from build123d import *

# Parameters (mm, degrees)
BOSS_EXTRUDE1_DEPTH   = 32
BOSS_EXTRUDE1_2_DEPTH = 32
BOSS_EXTRUDE2_DEPTH   = 72
CUT_EXTRUDE1_REACH    = 135.547
CUT_EXTRUDE2_REACH    = 168.292
SKETCH3_R             = 10


with BuildPart() as part:
    # Sketch1 → Boss-Extrude1 (new body)
    with BuildSketch(Plane.XY):
        Polygon((0, 42.5), (1.56434465, 52.376883406), (120.39128367, 33.556545174), (75, 85), (0, 85), align=None)
    extrude(amount=BOSS_EXTRUDE1_DEPTH)



with BuildPart() as body_2:
    # Sketch1 → Boss-Extrude1 2 (new body)
    with BuildSketch(Plane.XY):
        Polygon((150, 0), (120.39128367, 33.556545174), (118.82693902, 23.679661768), (0, 42.5), (0, 0), align=None)
    extrude(amount=BOSS_EXTRUDE1_2_DEPTH)


with BuildPart() as part_1:
    add(part.part)

    add(body_2.part)  # Boss-Extrude2 merges body 2
    # Sketch1<4> → Boss-Extrude2 (add)
    with BuildSketch(Plane.XY):
        Polygon((0, 42.5), (1.56434465, 52.376883406), (120.39128367, 33.556545174), (118.82693902, 23.679661768), align=None)
    extrude(amount=BOSS_EXTRUDE2_DEPTH)

    # Cut-Extrude1: up to this plane
    cut_extrude1_end = Plane(origin=(0, 0, 32), z_dir=(0, 1, 0))
    # Sketch2 → Cut-Extrude1 (cut, up to the surface)
    with BuildSketch(Plane(origin=(84.338521401, 74.416342412, 0), x_dir=(0, 0, -1), z_dir=(0.7498378553650925, 0.6616216370868464, 0)), mode=Mode.PRIVATE) as cut_extrude1_sk1:
        Polygon((0, -22.564325319), (-8, -22.564325319), (-8, -12.564325319), (-24, -12.564325319), (-24, -72.564325319), (-8, -72.564325319), (-8, -62.564325319), (0, -62.564325319), align=None)
    cut_extrude1_tool1 = split(extrude(cut_extrude1_sk1.sketch, amount=-CUT_EXTRUDE1_REACH, mode=Mode.PRIVATE), bisect_by=cut_extrude1_end, keep=Keep.BOTH, mode=Mode.PRIVATE)
    add(cut_extrude1_tool1.solids().sort_by_distance((112.5, 42.5, 13))[0], mode=Mode.SUBTRACT)

    # Sketch3 → Cut-Extrude2 (cut, up to next)
    with BuildSketch(Plane(origin=(6.56661113, 41.459950971, 0), x_dir=(0.9876883405951378, -0.1564344650402311, 0), z_dir=(-0.1564344650402311, -0.9876883405951378, 0)), mode=Mode.PRIVATE) as cut_extrude2_sk1:
        with Locations((43.351535236, 54)):
            Circle(SKETCH3_R)
    cut_extrude2_tool1 = extrude(cut_extrude2_sk1.sketch, amount=-CUT_EXTRUDE2_REACH, mode=Mode.PRIVATE) & part_1.part
    # Sketch3 → Cut-Extrude2 (cut, up to next)
    with BuildSketch(Plane(origin=(6.56661113, 41.459950971, 0), x_dir=(0.9876883405951378, -0.1564344650402311, 0), z_dir=(-0.1564344650402311, -0.9876883405951378, 0)), mode=Mode.PRIVATE) as cut_extrude2_sk2:
        Polygon((113.659666997, 72), (88.659666997, 72), (113.659666997, 47), align=None)
    cut_extrude2_tool2 = extrude(cut_extrude2_sk2.sketch, amount=-CUT_EXTRUDE2_REACH, mode=Mode.PRIVATE) & part_1.part
    # Sketch3 → Cut-Extrude2 (cut, up to next)
    with BuildSketch(Plane(origin=(6.56661113, 41.459950971, 0), x_dir=(0.9876883405951378, -0.1564344650402311, 0), z_dir=(-0.1564344650402311, -0.9876883405951378, 0)), mode=Mode.PRIVATE) as cut_extrude2_sk3:
        Polygon((-6.648464764, 72), (-6.648464764, 32), (16.445546003, 72), align=None)
    cut_extrude2_tool3 = extrude(cut_extrude2_sk3.sketch, amount=-CUT_EXTRUDE2_REACH, mode=Mode.PRIVATE) & part_1.part
    add(cut_extrude2_tool1.solids().sort_by_distance((49.384417, 34.678277, 54))[0], mode=Mode.SUBTRACT)
    add(cut_extrude2_tool2.solids().sort_by_distance((110.596203, 24.983282, 63.666667))[0], mode=Mode.SUBTRACT)
    add(cut_extrude2_tool3.solids().sort_by_distance((7.603228, 41.295767, 58.666667))[0], mode=Mode.SUBTRACT)


solid = part_1.part
Geometry: final body of the model. Coordinates: model frame, mm. A direction names the side the tool comes from. Coordinates: 2 decimals unless noted, no trailing zeros. Write each loop counter-clockwise with the first axis right and the second up, starting at its lowest first coordinate (ties: lowest second). Pieces come first, ordered by that corner, then holes. Notation, with made-up numbers: (65.25, 26.5) - (118.25, 26.5) arc R23 ccw to (118.25, 41.5) - close; hole circle Ø5 at (-2, 84.5). An arc over 180 degrees is marked (long way). Return JSON: item names as keys, results as strings.
Item 1: Section query D-D (z = 51). Output: boundary loops of the cut face in (x, y).
Completed:
{"outline": "(10.83, 40.78) - (39.96, 36.17) - (41.53, 46.05) - (12.4, 50.66) - close; (58.81, 33.19) - (114.88, 24.31) - (116.44, 34.18) - (60.37, 43.06) - close"}
Item 2: Pin query (flat end, axial travel): pin 1 Ø13 at (x, y) = (38, 14.5) entering from +Z; pin 2 Ø6 at (x, y) = (35.5, 11) entering from -Z; pin 3 Ø12 at (x, z) = (112, 48.5) entering from -Y; pin 4 Ø2 at (x, y) = (101.5, 33.5) entering from +Z. Return the tip coordinate at first contact, or that it passes through.
Completed:
{"pin 1": "stops at z = 32", "pin 2": "stops at z = 0", "pin 3": "stops at y = 23.82", "pin 4": "stops at z = 66.65"}
Item 3: Line query: L1, parallel to Z at x = 60, y = 32.5; L2, parallel to X at y = 17, z = 19.5; L3, parallel to Z at x = 29, y = 74. Output: solid intervals per line, ascending.
Completed:
{"L1": "z = 0 to 8, 24 to 32", "L2": "x = 0 to 38.26, 128.94 to 135", "L3": "z = 0 to 32"}
Item 4: Section query C-C (y = 17). Output: boundary loops of the cut face in (x, z).
Completed:
{"outline": "(0, 0) - (53.37, 0) - (53.37, 8) - (38.26, 8) - (38.26, 24) - (128.94, 24) - (128.94, 8) - (113.83, 8) - (113.83, 0) - (135, 0) - (135, 32) - (0, 32) - close"}
Item 5: Pull-direction query (X, two-part tool) for faces 1 (the face through (48.01, 39.89, 44.24)), 2 (the face through (67.14, 29.15, 3.94)), 3 (the face through (60, 38, 72)), 4 (the face through (119.62, 28.69, 39.39)); classes: +X half, -X half, draft (parallel to the pull), parting line (faces both ways), or undercut.
Completed:
{"face 1": "undercut", "face 2": "undercut", "face 3": "draft", "face 4": "+X half"}
Item 6: Reachability of faces 5 (the face through (56.336, 32.953, 15.888)), 6 (the face through (60.245, 32.958, 51.72)), 7 (the face through (60.146, 43.098, 47.276)), 8 (the face through (38, 85, 16)), 9 (the face through (121.17, 10.14, 16.11)) from +Z, -Z, +X, -X, +Y, -Y: full face, straight path, thin tool, end or side. Return the list, or none.
Completed:
{"face 5": "-Y", "face 6": "+Z, -X, -Y", "face 7": "+Z, +X, +Y", "face 8": "+Z, -Z, +X, -X, +Y", "face 9": "+Y"}
Item 7: Section query B-B (x = 122.5). Output: boundary loops of the cut face in (y, z), and give its area (3 significant figures).
Completed:
{"outline": "(0, 0) - (24.65, 0) - (24.65, 8) - (11.31, 8) - (11.31, 24) - (31.17, 24) - (31.17, 32) - (0, 32) - close", "area": "628 mm2"}
Item 8: Section query A-A (z = 12). Output: boundary loops of the cut face in (x, y), and give its area (3 significant figures).
Completed:
{"outline": "(0, 0) - (18.99, 0) - (92.65, 65) - (75, 85) - (0, 85) - close; (109.68, 0) - (150, 0) - (132.35, 20) - close", "area": "5,710 mm2"}
